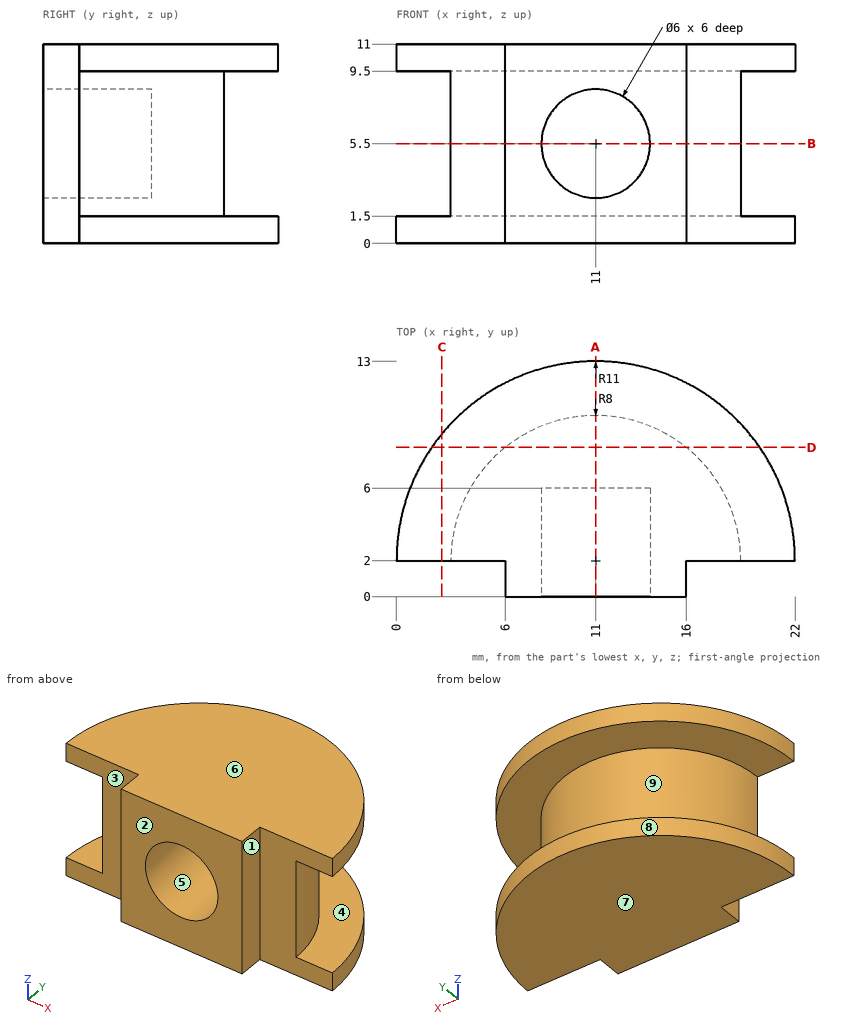
Geometry check sheet. Reference: drawing and pictorial views, mm from the part's lowest x, y, z. A direction names the side the tool comes from. Coordinates: 2 decimals unless noted, no trailing zeros. Loops run counter-clockwise (first coordinate to the right, second up) from the corner with the lowest first, then second, coordinate; pieces in that order, holes last. Notation, with made-up numbers: (50.25, -19.5) -> (84.25, -19.5) arc R14 cw to (84.25, -15.5) -> close; hole circle Ø7 at (25.5, 74.25). An arc over 180 degrees is marked (long way). Put each result on its own line as item: value.
1) Gauge pin test, flat ends, axial feed: pin 1 Ø1 at (y, z) = (1, 5) entering from -X; pin 2 Ø3 at (x, z) = (4, 8) entering from -Y; pin 3 Ø1.8 at (x, z) = (10.5, 4) entering from -Y; pin 4 Ø5 at (x, z) = (10, 1.5) entering from -Y. Record the tip position at first contact, or that the pin passes through.
Result set:
pin 1: stops at x = 6
pin 2: stops at y = 2
pin 3: stops at y = 6
pin 4: stops at y = 0
2) Cross-section at C-C on x = 2.5. Record the boundary of the cut face in (y, z).
Result set:
outline: (2, 0) -> (8.98, 0) -> (8.98, 1.5) -> (2, 1.5) -> close; (2, 9.5) -> (8.98, 9.5) -> (8.98, 11) -> (2, 11) -> close
3) Cross-section at A-A on x = 11. Record the boundary of the cut face in (y, z), plus the area to 3 significant figures.
Result set:
outline: (0, 0) -> (13, 0) -> (13, 1.5) -> (10, 1.5) -> (10, 9.5) -> (13, 9.5) -> (13, 11) -> (0, 11) -> (0, 8.5) -> (6, 8.5) -> (6, 2.5) -> (0, 2.5) -> close
area: 83.0 mm^2
4) Cross-section at B-B on z = 5.5. Record the boundary of the cut face in (x, y), plus the area to 3 significant figures.
Result set:
outline: (3, 2) -> (6, 2) -> (6, 0) -> (8, 0) -> (8, 6) -> (14, 6) -> (14, 0) -> (16, 0) -> (16, 2) -> (19, 2) arc R8 ccw to start
area: 84.5 mm^2
5) Tool access check on the marked faces 1, 2, 3, 4 and 5. Record the directions out of +Z, -Z, +X, -X, +Y, -Y that give a thin tool (end or side, any length) a straight path to the whole face; none if there is none.
Result set:
face 1: +Z, -Z, +X, -Y
face 2: +Z, -Z, +X, -X, -Y
face 3: +Z, -Z, -X, -Y
face 4: +Y
face 5: -Y
6) Release check for a two-part mould opening along Z. For the marked faces 6, 7, 8 and 9 record: released by +Z, released by -Z, zero draft, split by the parting line, or undercut.
Result set:
face 6: released by +Z
face 7: released by -Z
face 8: zero draft
face 9: undercut
7) Thickness scan on line 1 (Z direction, x = 6.25, y = 11.25); line 2 (X direction, y = 1.5, z = 5.5); line 3 (Z direction, x = 9, y = 4.25). Record the ranges inside material, lowest first.
Result set:
line 1: z = 0 to 1.5, 9.5 to 11
line 2: x = 6 to 8, 14 to 16
line 3: z = 0 to 3.26, 7.74 to 11
8) Cross-section at D-D on y = 8.25. Record the boundary of the cut face in (x, z), plus the area to 3 significant figures.
Result set:
outline: (1.95, 0) -> (20.05, 0) -> (20.05, 1.5) -> (15.99, 1.5) -> (15.99, 9.5) -> (20.05, 9.5) -> (20.05, 11) -> (1.95, 11) -> (1.95, 9.5) -> (6.01, 9.5) -> (6.01, 1.5) -> (1.95, 1.5) -> close
area: 134 mm^2
